Check sheet for the modelled part. Datum: model origin and axes. Units: mm. Face numbers are marked on the shaded views. A direction names the side the tool comes from. Round coordinates to 2 decimals unless told otherwise and drop trailing zeros. Write each loop counter-clockwise with the first axis right and the second up, starting at its lowest first coordinate (ties: lowest second). Pieces come first, ordered by that corner, then holes.
Item 1: Section check D-D, the plane x = 9. Record the cut outline in (y, z), plus the area to 3 significant figures.
Item 2: Release check for a two-part mould opening along Y. For the marked faces 1, 2, 3 and 4 record: pulls with the +Y half, pulls with the -Y half, needs draft (parallel to the pull), parting line crosses it, or undercut.
Item 3: Depth check by flat-ended pin: pin 1 (1.6 mm diameter, centred on y = -15, z = -10, fed in from +X); pin 2 (3.5 mm diameter, centred on y = -18.5, z = -15.5, fed in from -X); pin 3 (1.4 mm diameter, centred on x = 19.99, y = -18.79, fed in from +Z). Enter the tip coordinate at first touch or a pass-through.
Item 4: Section check C-C, the plane y = -8. Record the cut outline in (x, z).
Item 5: Set-up check for the marked faces 5, 6, 7 and 8: record each of +Z, -Z, +X, -X, +Y, -Y from which the full face is reachable in a straight line by a thin tool's end or side.
Item 6: Material ranges on line 1 along X through (y, z) = (-21, -18); line 2 along Z through (x, y) = (-12.5, -18); line 3 along X through (y, z) = (-8.5, -10.75), recorded low to high.
Item 7: Section check A-A, the plane y = 11.5. Record the cut outline in (x, z).
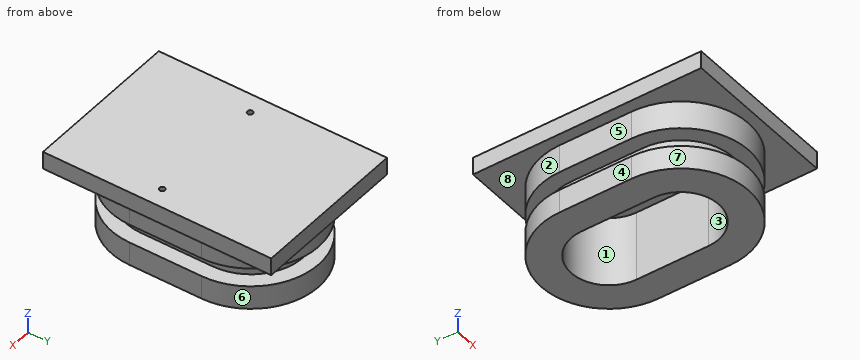
from build123d import *

# Parameters (mm, degrees)
SKETCH1_W                 = 45
SKETCH1_H                 = 65
BOSS_EXTRUDE1_DEPTH       = 5
BOSS_EXTRUDE2_DEPTH       = 20
BOSS_EXTRUDE3_DEPTH       = 5.3
M2X0_4_TAPPED_HOLE1_D     = 1.6
M2X0_4_TAPPED_HOLE1_DEPTH = 6
M2X0_4_TAPPED_HOLE1_TIP   = 0.480688495


with BuildPart() as part:
    # Sketch1 → Boss-Extrude1 (new body)
    with BuildSketch(Plane.XY):
        with Locations((2.886207951, -16.286739239)):
            Rectangle(SKETCH1_W, SKETCH1_H)
    extrude(amount=BOSS_EXTRUDE1_DEPTH)

    # Sketch4 → Boss-Extrude2 (add)
    with BuildSketch(Plane(origin=(0, 0, 0), x_dir=(-1, 0, 0), z_dir=(0, 0, -1))):
        with BuildLine():
            Line((16.363792049, -6.036739239), (16.363792049, -26.536739239))
            ThreePointArc((16.363792049, -26.536739239), (-2.886207951, -45.786739239), (-22.136207951, -26.536739239))
            Line((-22.136207951, -26.536739239), (-22.136207951, -6.036739239))
            ThreePointArc((-22.136207951, -6.036739239), (-2.886207951, 13.213260761), (16.363792049, -6.036739239))
        make_face()
        with BuildLine():
            Line((7.863792049, -6.036739239), (7.863792049, -26.536739239))
            ThreePointArc((7.863792049, -26.536739239), (-2.886207951, -37.286739239), (-13.636207951, -26.536739239))
            Line((-13.636207951, -26.536739239), (-13.636207951, -6.036739239))
            ThreePointArc((-13.636207951, -6.036739239), (-2.886207951, 4.713260761), (7.863792049, -6.036739239))
        make_face(mode=Mode.SUBTRACT)
    extrude(amount=BOSS_EXTRUDE2_DEPTH)


with BuildPart() as body_2:
    # Sketch6 → Boss-Extrude3 (new body)
    with BuildSketch(Plane(origin=(0, 0, 0), x_dir=(-1, 0, 0), z_dir=(0, 0, -1))):
        with BuildLine():
            Line((16.363792049, -6.036739239), (16.363792049, -26.536739239))
            ThreePointArc((16.363792049, -26.536739239), (-2.886207951, -45.786739239), (-22.136207951, -26.536739239))
            Line((-22.136207951, -26.536739239), (-22.136207951, -6.036739239))
            ThreePointArc((-22.136207951, -6.036739239), (-2.886207951, 13.213260761), (16.363792049, -6.036739239))
        make_face()
        with BuildLine():
            Line((12.029792049, -6.036739239), (12.029792049, -26.536739239))
            ThreePointArc((12.029792049, -26.536739239), (-2.886207951, -41.452739239), (-17.802207951, -26.536739239))
            Line((-17.802207951, -26.536739239), (-17.802207951, -6.036739239))
            ThreePointArc((-17.802207951, -6.036739239), (-2.886207951, 8.879260761), (12.029792049, -6.036739239))
        make_face(mode=Mode.SUBTRACT)
    extrude(amount=BOSS_EXTRUDE3_DEPTH)


with BuildPart() as body_2_1:
    # Body-Move/Copy1: read off the stored shape, not the designer's step
    # Body-Move/Copy1: moved
    add(body_2.part.moved(Location((0, 0, -8))))


with BuildPart() as part_1:
    add(part.part)

    # Combine1: cut body 2
    add(body_2_1.part, mode=Mode.SUBTRACT)

    # M2x0.4 Tapped Hole1
    with Locations(Plane.XY.offset(5)):
        with Locations((-14.213792049, -18.786739239), (19.986207951, -18.786739239)):
            Hole(M2X0_4_TAPPED_HOLE1_D / 2, depth=M2X0_4_TAPPED_HOLE1_DEPTH)
            with Locations((0, 0, -(M2X0_4_TAPPED_HOLE1_DEPTH + M2X0_4_TAPPED_HOLE1_TIP / 2))):  # 118° drill point
                Cone(0, M2X0_4_TAPPED_HOLE1_D / 2, M2X0_4_TAPPED_HOLE1_TIP, mode=Mode.SUBTRACT)


solid = part_1.part
Values found:
1. outline: (-48.79, 0) - (-44.79, 0) - (-44.79, -8) - (-40.14, -8) - (-40.14, -13.3) - (-44.79, -13.3) - (-44.79, -20) - (-35.38, -20) - (-35.38, 0) - (2.81, 0) - (2.81, -20) - (12.22, -20) - (12.22, -13.3) - (7.57, -13.3) - (7.57, -8) - (12.22, -8) - (12.22, 0) - (16.21, 0) - (16.21, 5) - (-48.79, 5) - close
1. area: 652 mm2
2. face 1: undercut
2. face 2: pulls with the +Y half
2. face 3: undercut
2. face 4: needs draft
3. pin 1: stops at x = 17.8
3. pin 2: stops at x = -16.36
3. pin 3: stops at z = -1.06
4. outline: (-19.61, 0) - (-16.36, 0) - (-16.36, -8) - (-12.03, -8) - (-12.03, -13.3) - (-16.36, -13.3) - (-16.36, -20) - (-7.86, -20) - (-7.86, 0) - (13.64, 0) - (13.64, -20) - (22.14, -20) - (22.14, -13.3) - (17.8, -13.3) - (17.8, -8) - (22.14, -8) - (22.14, 0) - (25.39, 0) - (25.39, 5) - (-19.61, 5) - close
5. face 5: -Z, -X, +Y, -Y
5. face 6: -Z, +Y
5. face 7: -Z, -Y
5. face 8: -Z
6. line 1: x = -16.36 to -7.86, 13.64 to 22.14
6. line 2: z = -20 to -13.3, -8 to 5
6. line 3: x = -12.03 to -7.86, 13.64 to 17.8
7. outline: (-19.61, 0) - (-5.05, 0) - (-5.05, -8) - (10.83, -8) - (10.83, 0) - (25.39, 0) - (25.39, 5) - (-19.61, 5) - close; (-5.05, -20) - (10.83, -20) - (10.83, -13.3) - (-5.05, -13.3) - close
